```python
from build123d import *

# Parameters (mm, degrees)
F0_R     = 25.4
F0_R_2   = 3.5
F1_DEPTH = 2.5


with BuildPart() as f1:
    # F0 (on Top) → F1 (new body, symmetric)
    with BuildSketch(Plane.XY):
        Circle(F0_R)
        with BuildLine():
            ThreePointArc((-4.520769, -19.810731), (-5.867147, -18.750304), (-5.898131, -17.036747))
            Line((-5.898131, -17.036747), (-2.335578, -9.159014))
            ThreePointArc((-2.335578, -9.159014), (-1.55413, -8.27532), (-0.41057, -7.98576))
            ThreePointArc((-0.41057, -7.98576), (0, -7.996308), (0.41057, -7.98576))
            ThreePointArc((0.41057, -7.98576), (1.55413, -8.27532), (2.335578, -9.159014))
            Line((2.335578, -9.159014), (5.898131, -17.036747))
            ThreePointArc((5.898131, -17.036747), (5.867147, -18.750304), (4.520769, -19.810731))
            ThreePointArc((4.520769, -19.810731), (0, -20.32), (-4.520769, -19.810731))
        make_face(mode=Mode.SUBTRACT)
        with BuildLine():
            ThreePointArc((-18.307306, -8.817309), (-18.317684, -7.103503), (-16.997289, -6.010894))
            Line((-16.997289, -6.010894), (-8.617015, -3.884523))
            ThreePointArc((-8.617015, -3.884523), (-7.43889, -3.94451), (-6.499505, -4.658044))
            ThreePointArc((-6.499505, -4.658044), (-6.251765, -4.985616), (-5.987533, -5.300037))
            ThreePointArc((-5.987533, -5.300037), (-5.500922, -6.374646), (-5.704596, -7.53658))
            Line((-5.704596, -7.53658), (-9.642441, -15.233582))
            ThreePointArc((-9.642441, -15.233582), (-11.001472, -16.277743), (-12.669999, -15.886268))
            ThreePointArc((-12.669999, -15.886268), (-15.886816, -12.669313), (-18.307306, -8.817309))
        make_face(mode=Mode.SUBTRACT)
        Circle(F0_R_2, mode=Mode.SUBTRACT)
        with BuildLine():
            ThreePointArc((12.669999, -15.886268), (11.001472, -16.277743), (9.642441, -15.233582))
            Line((9.642441, -15.233582), (5.704596, -7.53658))
            ThreePointArc((5.704596, -7.53658), (5.500922, -6.374646), (5.987533, -5.300037))
            ThreePointArc((5.987533, -5.300037), (6.251765, -4.985616), (6.499505, -4.658044))
            ThreePointArc((6.499505, -4.658044), (7.43889, -3.94451), (8.617015, -3.884523))
            Line((8.617015, -3.884523), (16.997289, -6.010894))
            ThreePointArc((16.997289, -6.010894), (18.317684, -7.103503), (18.307306, -8.817309))
            ThreePointArc((18.307306, -8.817309), (15.886816, -12.669313), (12.669999, -15.886268))
        make_face(mode=Mode.SUBTRACT)
        with BuildLine():
            ThreePointArc((-18.308068, 8.815727), (-16.974632, 9.89238), (-15.297143, 9.541285))
            Line((-15.297143, 9.541285), (-8.409663, 4.315093))
            ThreePointArc((-8.409663, 4.315093), (-7.722014, 3.356597), (-7.69418, 2.177275))
            ThreePointArc((-7.69418, 2.177275), (-7.795824, 1.779346), (-7.876901, 1.376723))
            ThreePointArc((-7.876901, 1.376723), (-8.413667, 0.326267), (-9.449094, -0.238948))
            Line((-9.449094, -0.238948), (-17.922058, -1.959219))
            ThreePointArc((-17.922058, -1.959219), (-19.585758, -1.54771), (-20.32, 0.000878))
            ThreePointArc((-20.32, 0.000878), (-19.810535, 4.521625), (-18.308068, 8.815727))
        make_face(mode=Mode.SUBTRACT)
        with BuildLine():
            ThreePointArc((-1.869664, 9.265356), (-2.190304, 8.130118), (-3.094981, 7.373061))
            ThreePointArc((-3.094981, 7.373061), (-3.469468, 7.204424), (-3.834802, 7.016782))
            ThreePointArc((-3.834802, 7.016782), (-4.99075, 6.781494), (-6.078231, 7.238617))
            Line((-6.078231, 7.238617), (-12.706, 12.790476))
            ThreePointArc((-12.706, 12.790476), (-13.421569, 14.34778), (-12.668626, 15.887363))
            ThreePointArc((-12.668626, 15.887363), (-8.816518, 18.307687), (-4.522481, 19.81034))
            ThreePointArc((-4.522481, 19.81034), (-2.849335, 19.4391), (-2.077936, 17.908682))
            Line((-2.077936, 17.908682), (-1.869664, 9.265356))
        make_face(mode=Mode.SUBTRACT)
        with BuildLine():
            ThreePointArc((20.32, 0.000878), (19.585758, -1.54771), (17.922058, -1.959219))
            Line((17.922058, -1.959219), (9.449094, -0.238948))
            ThreePointArc((9.449094, -0.238948), (8.413667, 0.326267), (7.876901, 1.376723))
            ThreePointArc((7.876901, 1.376723), (7.795824, 1.779346), (7.69418, 2.177275))
            ThreePointArc((7.69418, 2.177275), (7.722014, 3.356597), (8.409663, 4.315093))
            Line((8.409663, 4.315093), (15.297143, 9.541285))
            ThreePointArc((15.297143, 9.541285), (16.974632, 9.89238), (18.308068, 8.815727))
            ThreePointArc((18.308068, 8.815727), (19.810535, 4.521625), (20.32, 0.000878))
        make_face(mode=Mode.SUBTRACT)
        with BuildLine():
            ThreePointArc((3.094981, 7.373061), (2.190304, 8.130118), (1.869664, 9.265356))
            Line((1.869664, 9.265356), (2.077936, 17.908682))
            ThreePointArc((2.077936, 17.908682), (2.849335, 19.4391), (4.522481, 19.81034))
            ThreePointArc((4.522481, 19.81034), (8.816518, 18.307687), (12.668626, 15.887363))
            ThreePointArc((12.668626, 15.887363), (13.421569, 14.34778), (12.706, 12.790476))
            Line((12.706, 12.790476), (6.078231, 7.238617))
            ThreePointArc((6.078231, 7.238617), (4.99075, 6.781494), (3.834802, 7.016782))
            ThreePointArc((3.834802, 7.016782), (3.469468, 7.204424), (3.094981, 7.373061))
        make_face(mode=Mode.SUBTRACT)
    extrude(amount=F1_DEPTH, both=True)

    # F2 (on Right) → F3 (revolve, cut)
    with BuildSketch(Plane.YZ):
        Polygon((25.408719, -1.552115), (25.503, 0), (24.003, 0), align=None)
        Polygon((24.003, 0), (25.503, 0), (25.408719, 1.552115), align=None)
    revolve(axis=Axis((0, 0, 1.759876), (0, 0, 1)), mode=Mode.SUBTRACT)


solid = f1.part
```
For this review, take the finished solid that the model builds, in its own axes (mm). A direction names the side the tool comes from. Give positions to 0.01 mm unless a question says otherwise; leave off trailing zeros.
1) For faces 3 (the face through (13.7, -1.1, 0)), 4 (the face through (0, -5, 2.5)), list the 3-axis set-ups (+Z, -Z, +X, -X, +Y, -Y) from which the entire face can be reached by the end or side of a thin tool; tool diameter is ignored.
2) Wall thickness on line 1 (Y direction, x = -14.5, z = -1.7); line 2 (X direction, y = 12.5, z = 1.9); line 3 (Y direction, x = -11.5, z = 0.55): over which ranges is each line inside the solid? List them lowest first.
3) Insertion check: pin 1 (1 mm diameter, centred on y = -17.5, z = 0.5, fed in from -X); pin 2 (2 mm diameter, centred on y = -2, z = 1, fed in from -X); pin 3 (1.5 mm diameter, centred on y = -20, z = -1, fed in from +X). Each pin has a flat end and moves straight along its axis. Give the tip position at first contact, or say it passes through.
4) The part is to be moulded in two halves that separate along X. For faces 1 (the face through (0, -5, -2.5)), 2 (the face through (-4.97, 6.78, 0.04)), say which applies: released by +X, released by -X, zero draft, split by the parting line, or undercut.
5) Take a section at A-A (z = -0.9). State how many separate pieces and enclosed holes the cut face has, then the cut area to 3 significant figures.
Derived:
1. face 3: +Z, -Z
1. face 4: +Z, +X, -X, +Y, -Y
2. line 1: y = -20.85 to -14.24, -5.38 to -1.26, 8.94 to 20.85
2. line 2: x = -22.11 to -12.36, -1.95 to 1.95, 12.36 to 22.11
2. line 3: y = -21.63 to -16.32, -4.62 to -0.66, 6.66 to 11.78, 16.75 to 21.63
3. pin 1: stops at x = -17.89
3. pin 2: stops at x = -25.37
3. pin 3: stops at x = 16.3
4. face 1: zero draft
4. face 2: undercut
5. separate pieces: 1
5. enclosed holes: 8
5. area: 1,170 mm2
